Autodesk Inventor part; units mm, degrees
ref_plane "YZ Plane" through (0, 0, 0) normal (1, 0, 0) x (0, 1, 0)
ref_plane "XZ Plane" through (0, 0, 0) normal (0, 1, 0) x (-1, 0, 0)
ref_plane "XY Plane" through (0, 0, 0) normal (0, 0, 1) x (1, 0, 0)
sketch "Sketch1" plane through (0, 0, 0) normal (0, 0, 1) x (1, 0, 0)
  line L0 (38.0718, -21.4) -> (37, -25.4)
  line L1 (37, -25.4) -> (38.0718, -21.4)
  line L2 (8.9282, -21.4) -> (38.0718, -21.4)
  line L3 (38.0718, -21.4) -> (8.9282, -21.4)
  line L4 (10, -25.4) -> (8.9282, -21.4)
  line L5 (8.9282, -21.4) -> (10, -25.4)
  line L6 (10, -25.4) -> (0, -25.4)
  line L7 (10, -25.4) -> (0, -25.4)
  line L8 (47, -25.4) -> (37, -25.4)
  line L9 (37, -25.4) -> (47, -25.4)
  line L10 (38.0718, -21.4) -> (37, -25.4)
  line L11 (37, -25.4) -> (38.0718, -21.4)
  line L12 (8.9282, -21.4) -> (38.0718, -21.4)
  line L13 (38.0718, -21.4) -> (8.9282, -21.4)
  line L14 (10, -25.4) -> (8.9282, -21.4)
  line L15 (8.9282, -21.4) -> (10, -25.4)
  line L16 (10, -25.4) -> (0, -25.4)
  line L17 (10, -25.4) -> (0, -25.4)
  line L18 (47, -25.4) -> (37, -25.4)
  line L19 (37, -25.4) -> (47, -25.4)
  line L20 (0, -38.1) -> (47, -38.1)
  line L21 (47, -25.4) -> (72.4, -25.4)
  line L22 (72.4, -25.4) -> (72.4, -38.1)
  line L23 (72.4, -38.1) -> (47, -38.1)
  line L24 (0, -25.4) -> (-25.4, -25.4)
  line L25 (-25.4, -25.4) -> (-25.4, -38.1)
  line L26 (-25.4, -38.1) -> (0, -38.1)
  point P0 (0, 0)
  point P1 (0, 0)
  point P2 (0, 0)
  dimension "d52" = 4
  dimension "d53" = 27
  dimension "d54" = 29.1436
extrude "Extrusion1" add sketch "Sketch1" along normal blind 331
sketch "Sketch4" plane through (0, 0, 0) normal (0, 0, -1) x (-1, 0, 0)
  line L0 (-38.0718, -21.4) -> (-8.9282, -21.4)
  line L1 (-8.9282, -21.4) -> (-8.9282, -38.1)
  line L2 (25.4, -38.1) -> (-72.4, -38.1)
  line L3 (25.4, -38.1) -> (25.4, -40.45)
  line L4 (25.4, -40.45) -> (-72.4, -40.45)
  line L5 (-72.4, -40.45) -> (-72.4, -38.1)
  line L6 (-72.4, -38.1) -> (25.4, -38.1)
  line L7 (25.4, -38.1) -> (25.4, -40.45)
  point P0 (0, 0)
  dimension "d26" = 2.35
extrude "Extrusion4" add sketch "Sketch4" against normal blind 331
sketch "Sketch3" plane through (37, -25.4, 331) normal (0, 1, 0) x (1, 0, 0)
  line L0 (35.4, 0) -> (0, 0)
  line L1 (-28.0718, 0) -> (-27, 0)
  line L2 (0, 0) -> (-27, 0)
  line L3 (-27, 0) -> (-13.5, 0)
  line L4 (-13.5, 0) -> (-13.5, 11.6369)
  line L5 (-13.5, 0) -> (-1.8631, 0) construction
  line L6 (35.4, 0) -> (25.4, 0)
  line L7 (25.4, 0) -> (25.4, 25)
  line L8 (25.4, 25) -> (25.4, 75)
  line L9 (25.4, 75) -> (25.4, 125)
  line L10 (25.4, 125) -> (25.4, 175)
  line L11 (25.4, 175) -> (25.4, 225)
  line L12 (25.4, 225) -> (25.4, 275)
  line L13 (25.4, 275) -> (25.4, 325)
  circle A0 centre (25.4, 325) radius 3.175
  circle A1 centre (25.4, 275) radius 3.175
  circle A2 centre (25.4, 225) radius 3.175
  circle A3 centre (25.4, 175) radius 3.175
  circle A4 centre (25.4, 125) radius 3.175
  circle A5 centre (25.4, 75) radius 3.175
  circle A6 centre (25.4, 25) radius 3.175
  circle A7 centre (-52.4, 325) radius 3.175
  circle A8 centre (-52.4, 275) radius 3.175
  circle A9 centre (-52.4, 225) radius 3.175
  circle A10 centre (-52.4, 175) radius 3.175
  circle A11 centre (-52.4, 125) radius 3.175
  circle A12 centre (-52.4, 75) radius 3.175
  circle A13 centre (-52.4, 25) radius 3.175
  point P0 (-37, 331)
  dimension "d8" = 90
  dimension "d9" = 10
  dimension "d10" = 25
  dimension "d11" = 50
  dimension "d12" = 50
  dimension "d13" = 50
  dimension "d14" = 50
  dimension "d15" = 50
  dimension "d16" = 50
  dimension "d17" = 6.35
  dimension "d18" = 6.35
  dimension "d19" = 6.35
  dimension "d20" = 6.35
  dimension "d21" = 6.35
  dimension "d22" = 6.35
  dimension "d23" = 6.35
extrude "Extrusion3" cut sketch "Sketch3" against normal blind 300
sketch "Sketch5" plane through (0, 0, 331) normal (0, 0, 1) x (1, 0, 0)
  line L0 (37, -25.4) -> (38.0718, -21.4)
  line L1 (38.0718, -21.4) -> (72.4488, -21.4)
  line L2 (72.4488, -40.7637) -> (72.4488, -13.0005)
  line L3 (-25.4, -25.4) -> (-25.4, -40.45)
  line L4 (72.4488, -21.4) -> (-25.4, -21.4)
  line L5 (-25.4, -21.4) -> (-25.4, -40.45)
  line L6 (-25.4, -40.45) -> (72.4488, -40.45)
  line L7 (72.4488, -40.45) -> (72.4488, -21.4)
  point P0 (0, 0)
extrude "Extrusion5" add sketch "Sketch5" along normal blind 35
sketch "Sketch6" plane through (0, 0, 366) normal (0, 0, 1) x (1, 0, 0)
  point P0 (0, 0)
sketch "Sketch7" plane through (72.4, -40.45, 0) normal (1, 0, 0) x (0, 0, -1)
  point P0 (0, 40.45)
sketch "Sketch8" plane through (0, 0, 366) normal (0, 0, 1) x (1, 0, 0)
  line L0 (-25.4, -21.4) -> (-25.4, -40.45)
  line L1 (-25.4, -21.4) -> (-25.4, -25.4)
  line L2 (72.4, -40.45) -> (72.4488, -40.45)
  line L3 (-25.4, -25.4) -> (72.4488, -40.45)
  line L4 (72.4, -40.45) -> (72.4, -25.4)
  line L5 (72.4488, -40.45) -> (72.4, -25.4)
  line L6 (72.4, -25.4) -> (-25.4, -40.45)
  line L7 (23.5, -32.925) -> (-0.95, -32.925)
  line L8 (-0.95, -32.925) -> (47.95, -32.925)
  circle A0 centre (-0.95, -32.925) radius 2.5
  circle A1 centre (23.5, -33.0837) radius 2.5
  circle A2 centre (47.95, -32.925) radius 2.5
  point P0 (0, 0)
  point P1 (-25.4, -38.1)
  dimension "d31" = 4
  dimension "d32" = 24.45
  dimension "d33" = 48.9
  dimension "d34" = 5
  dimension "d35" = 5
  dimension "d36" = 5
extrude "Extrusion6" cut sketch "Sketch8" against normal blind 30 contours A0 | A1 L6 L3 | L3 L7 A1 | A1 L7 L6 | L6 L3 A1 | A1 L8 L6 | A2 | L3 L8 A1
sketch "Sketch9" plane through (0, 0, 366) normal (0, 0, 1) x (1, 0, 0)
  circle A0 centre (-0.95, -32.925) radius 2.5
  line L0 (-0.95, -32.925) -> (13.1454, -27.7947)
  line L1 (-0.95, -32.925) -> (14.05, -32.925) construction
  line L2 (-0.95, -32.925) -> (-15.0454, -27.7947)
  line L3 (-0.95, -32.925) -> (14.05, -32.925) construction
  circle A1 centre (47.95, -32.925) radius 2.5
  line L4 (47.95, -32.925) -> (62.0454, -27.7947)
  line L5 (47.95, -32.925) -> (62.95, -32.925) construction
  circle A2 centre (-15.0454, -27.7947) radius 2.5
  circle A3 centre (62.0454, -27.7947) radius 2.5
  point P0 (0, 0)
  dimension "d39" = 15
  dimension "d40" = 20
  dimension "d41" = 15
  dimension "d42" = 160
  dimension "d43" = 15
  dimension "d44" = 20
  dimension "d45" = 5
  dimension "d46" = 5
extrude "Extrusion7" cut sketch "Sketch9" against normal blind 30 contours A2 | A3
sketch "Sketch10" plane through (8.9282, -21.4, 0) normal (0, 1, 0) x (1, 0, 0)
  line L0 (-34.3282, -331) -> (-34.3282, -366)
  line L1 (63.5206, -331) -> (63.5206, -366)
  line L2 (-34.3282, -366) -> (63.5206, -366)
  line L3 (63.5206, -366) -> (63.5206, -331)
  line L4 (63.5206, -331) -> (-34.3282, -331)
  line L5 (-34.3282, -331) -> (-34.3282, -366)
  line L6 (63.4718, 0) -> (63.4718, -331)
  line L7 (63.4718, -331) -> (-34.3282, -331)
  line L8 (-34.3282, -331) -> (-34.3282, -346)
  line L9 (-34.3282, -346) -> (63.4718, -346)
  line L10 (63.4718, -346) -> (63.4718, -331)
  point P0 (-8.9282, 0)
  point P1 (-34.3282, -346)
  dimension "d49" = 15
extrude "Extrusion8" cut sketch "Sketch10" against normal blind 30 contours L9 L10 L4 L1 L2 L0
properties part number "5212_Bias_TxRx_Relative_Dovetail_Male_MPSv2_v3" material "Polyethylene, High Density"
Could you check a few things on this model? Use its own coordinates, in mm. Coordinates: 2 decimals unless noted, no trailing zeros. Order: outer loops, then holes, each group sorted by start corner. A loop starts at its lowest first (then second) coordinate and runs counter-clockwise, first axis right, second up. Notation, with made-up numbers: M 28,0.25 L 57,0.25 A23 ccw 57,38.25 Z; hole C 56,73 d7. An arc over 180 degrees is marked long. Use a Markdown table: item, result. Add a question column.
Q1. I want a section at A-A on z = 6. List the corners of the cut face in (x, y) for me (3 decimals).
Q2. I want a section at C-C on x = -8.5. List the corners of the cut face in (y, z) for me, then the cut area to 3 significant figures.
Q3. We'd pull the mould along X, two halves only. Please class faces 1 (the cylindrical face through (59.23, -32.82, 5.86)), 2 (the flat face through (-7, -25.4, 163)), 3 (the flat face through (-25.4, -33, 171)): pulls with the +X half, pulls with the -X half, needs draft (parallel to the pull), parting line crosses it, or undercut.
Q4. I want a section at B-B on z = 93. List the corners of the cut face in (x, y) for me, then the cut area to 3 significant figures.
Q5. I'm going to push flat-ended pins straight in: pin 1 (1.5 mm diameter, centred on x = 60, z = 157.5, fed in from +Y); pin 2 (5.5 mm diameter, centred on x = 62.4, z = 56, fed in from -Y); pin 3 (1.5 mm diameter, centred on x = 62, y = -29, fed in from +Z). Where does each tip first touch, or does it pass through?
Q6. If I drill on L1, parallel to X at y = -30.5, z = 56 (3 decimals); L2, parallel to Y at x = 58.5, z = 20.5; L3, parallel to Z at x = 22, y = -34.75, over which ranges is the centre line in solid material (lowest first)?
Checked values:
| question | item | result |
|---|---|---|
| 1 | outline | M -25.4,-40.45 L -18.575,-40.45 L -18.575,-25.4 L -25.4,-25.4 Z; M -12.225,-40.45 L 59.225,-40.45 L 59.225,-25.4 L 37,-25.4 L 38.072,-21.4 L 8.928,-21.4 L 10,-25.4 L -12.225,-25.4 Z; M 65.575,-40.45 L 72.4,-40.45 L 72.4,-25.4 L 65.575,-25.4 Z |
| 2 | outline | M -40.45,0 L -25.4,0 L -25.4,331 L -21.4,331 L -21.4,346 L -40.45,346 Z |
| 2 | area | 5,270 mm² |
| 3 | face 1 | undercut |
| 3 | face 2 | needs draft |
| 3 | face 3 | pulls with the -X half |
| 4 | outline | M -25.4,-40.45 L 72.4,-40.45 L 72.4,-25.4 L 37,-25.4 L 38.07,-21.4 L 8.93,-21.4 L 10,-25.4 L -25.4,-25.4 Z |
| 4 | area | 1,580 mm² |
| 5 | pin 1 | y = -25.4 |
| 5 | pin 2 | through |
| 5 | pin 3 | z = 336 |
| 6 | L1 | -25.4 to -18.575, -12.225 to 59.225, 65.575 to 72.4 |
| 6 | L2 | -40.45 to -25.4 |
| 6 | L3 | 0 to 336 |
